```python
from build123d import *

# Parameters (mm, degrees)
BOSS_EXTRUDE1_DEPTH = 24
BOSS_EXTRUDE2_DEPTH = 10


with BuildPart() as part:
    # Sketch1 → Boss-Extrude1 (new body)
    with BuildSketch(Plane(origin=(0, 0, 0), x_dir=(1, 0, 0), z_dir=(0, 1, 0))):
        Polygon((-24, 12), (0, 12), (0, -12), (-6, -12), (-6, 4), (-18, 4), (-18, -12), (-24, -12), align=None)
    extrude(amount=BOSS_EXTRUDE1_DEPTH)

    # Sketch1_3 → Boss-Extrude2 (add)
    with BuildSketch(Plane(origin=(0, 0, 0), x_dir=(1, 0, 0), z_dir=(0, 1, 0))):
        with BuildLine():
            ThreePointArc((20, 12), (32, 0), (20, -12))
            Line((20, -12), (0, -12))
            Line((0, -12), (0, 12))
            Line((0, 12), (20, 12))
        make_face()
        with BuildLine():
            ThreePointArc((12, 4), (8, 0), (12, -4))
            Line((12, -4), (20, -4))
            ThreePointArc((20, -4), (24, 0), (20, 4))
            Line((20, 4), (12, 4))
        make_face(mode=Mode.SUBTRACT)
    extrude(amount=BOSS_EXTRUDE2_DEPTH)


solid = part.part
```
The listing builds one solid part. Answer for the finished solid, in the listing's coordinates (mm). A direction names the side the tool comes from. Round coordinates to 2 decimals unless told otherwise and drop trailing zeros. Loops run counter-clockwise (first coordinate to the right, second up) from the corner with the lowest first, then second, coordinate; pieces in that order, holes last.
Q1. Section B-B, the plane z = 0 is taken. Determine the outline of the cut face in (x, y).
Q2. For a pull along X with two mould halves and no side action, classify faces 1 (the face through (-12, 12, -4)), 2 (the face through (32, 5, 0)), 3 (the face through (-12, 24, -6)) as released by +X, released by -X, zero draft, split by the parting line, or undercut.
Q3. Which of the six approach directions +Z, -Z, +X, -X, +Y, -Y give full straight-line access (tool end or side, diameter ignored) to faces 4 (the face through (-21, 12, 12)), 5 (the face through (-18, 12, 4)), 6 (the face through (-24, 12, 0)), 7 (the face through (0, 17, 0)), 8 (the face through (8, 5, 0))?
Q4. Find the intervals of material crossed by line 1 (X direction, y = 18, z = 10.75); line 2 (X direction, y = 9.75, z = -3.25); line 3 (X direction, y = 3, z = 3.5), in increasing order.
Q5. Section D-D, the plane y = 16.5 is taken. Determine the outline of the cut face in (x, z).
Q6. Section C-C, the plane z = 9 is taken. Determine the outline of the cut face in (x, y).
Q7. Given pin 1 Ø5 at (x, z) = (12, -7.5) entering from +Y; pin 2 Ø4 at (x, z) = (24.5, -4.5) entering from -Y; pin 3 Ø1.5 at (y, z) = (2.5, 9.5) entering from +X; pin 4 Ø4 at (y, z) = (21, -2.5) entering from +X, each flat-ended and moving along its own axis, determine where each tip first touches the part or whether it passes through.
Q8. Section A-A, the plane x = 16 is taken. Determine the outline of the cut face in (y, z), then the cut area to 3 significant figures.
Completed:
1. outline: (-24, 0) - (-18, 0) - (-18, 24) - (-24, 24) - close; (-6, 0) - (8, 0) - (8, 10) - (0, 10) - (0, 24) - (-6, 24) - close; (24, 0) - (32, 0) - (32, 10) - (24, 10) - close
2. face 1: undercut
2. face 2: released by +X
2. face 3: zero draft
3. face 4: +Z, +X, -X, +Y, -Y
3. face 5: +Z, +Y, -Y
3. face 6: +Z, -Z, -X, +Y, -Y
3. face 7: +Z, -Z, +X, +Y
3. face 8: +Y, -Y
4. line 1: x = -24 to -18, -6 to 0
4. line 2: x = -24 to -18, -6 to 9.67, 22.33 to 31.55
4. line 3: x = -24 to -18, -6 to 10.06, 21.94 to 31.48
5. outline: (-24, -12) - (0, -12) - (0, 12) - (-6, 12) - (-6, -4) - (-18, -4) - (-18, 12) - (-24, 12) - close
6. outline: (-24, 0) - (-18, 0) - (-18, 24) - (-24, 24) - close; (-6, 0) - (27.94, 0) - (27.94, 10) - (0, 10) - (0, 24) - (-6, 24) - close
7. pin 1: stops at y = 10
7. pin 2: stops at y = 0
7. pin 3: stops at x = 28.21
7. pin 4: stops at x = 0
8. outline: (0, -12) - (10, -12) - (10, -4) - (0, -4) - close; (0, 4) - (10, 4) - (10, 12) - (0, 12) - close
8. area: 160 mm2
